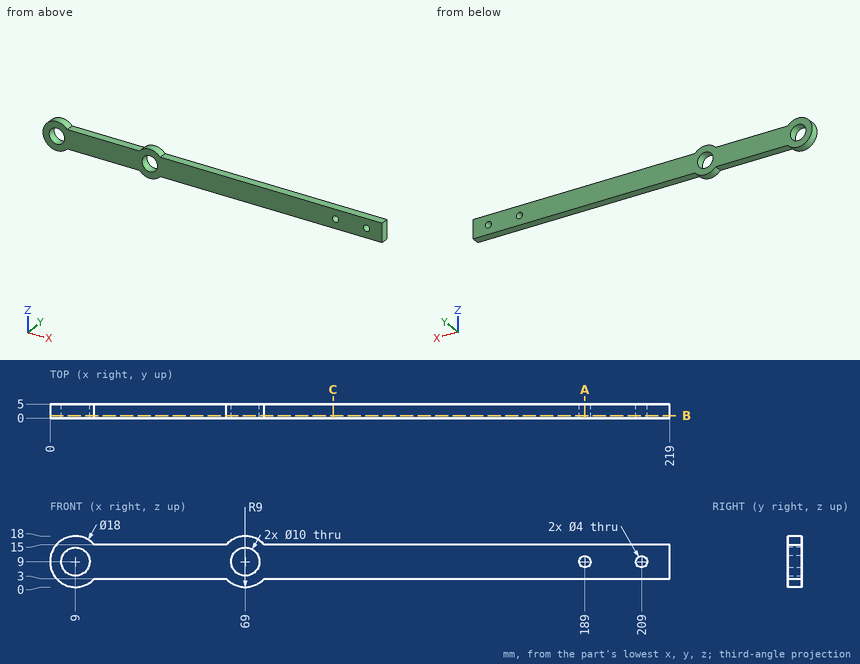
Could you check a few things on this drawing? It's one solid part, dimensions in mm from its lowest x, y, z. Give positions to 0.01 mm unless a question says otherwise; leave off trailing zeros. Loops run counter-clockwise (first coordinate to the right, second up) from the corner with the lowest first, then second, coordinate; pieces in that order, holes last. Notation, with made-up numbers: M -33.75,13 L 17.25,13 A16 ccw 17.25,43 Z; hole C 50,72.25 d10. An arc over 180 degrees is marked long. Return JSON: item names as keys, results as strings.
Item 1: Please list where these lines run through material, in increasing order: line 1 (X direction, y = 2.4, z = 9); line 2 (Z direction, x = 209, y = 1.9); line 3 (X direction, y = 2, z = 10.25).
A:
{"line 1": "x = 0 to 4, 14 to 64, 74 to 187, 191 to 207, 211 to 219", "line 2": "z = 3 to 7, 11 to 15", "line 3": "x = 0.09 to 4.16, 13.84 to 64.16, 73.84 to 187.44, 190.56 to 207.44, 210.56 to 219"}
Item 2: Imagine slicing it at A-A on x = 189. List the corners of the cut face in (y, z) for me.
A:
{"outline": "M 0,3 L 5,3 L 5,7 L 0,7 Z; M 0,11 L 5,11 L 5,15 L 0,15 Z"}
Item 3: I'm going to push flat-ended pins straight in: pin 1 Ø1 at (y, z) = (4, 3.5) entering from -X; pin 2 Ø2.5 at (x, y) = (142.5, 2) entering from -Z; pin 3 Ø3 at (x, z) = (189, 9) entering from +Y; pin 4 Ø1 at (x, y) = (34.5, 4.5) entering from +Z. Where does each tip first touch, or does it pass through?
A:
{"pin 1": "stops at x = 1.52", "pin 2": "stops at z = 3", "pin 3": "passes through", "pin 4": "stops at z = 15"}
Item 4: Imagine slicing it at C-C on x = 100. List the corners of the cut face in (y, z) for me, then the cut area to 3 significant figures.
A:
{"outline": "M 0,3 L 5,3 L 5,15 L 0,15 Z", "area": "60.0 mm^2"}
Item 5: Imagine slicing it at B-B on y = 0.85. List the corners of the cut face in (x, z) for me.
A:
{"outline": "M 15.71,3 L 62.29,3 A9 ccw 75.71,3 L 219,3 L 219,15 L 75.71,15 A9 ccw 62.29,15 L 15.71,15 A9 ccw long Z; hole C 9,9 d10; hole C 69,9 d10; hole C 189,9 d4; hole C 209,9 d4"}
